Read the model definition and answer for the solid it produces. Units are mm, in the model's axes. Face numbers are marked on the shaded views. A direction names the side the tool comes from. Give positions to 0.01 mm unless a question says otherwise; leave off trailing zeros. Write each loop counter-clockwise with the first axis right and the second up, starting at its lowest first coordinate (ties: lowest second). Pieces come first, ordered by that corner, then holes. Notation, with made-up numbers: M 61,23 L 93,23 A18 ccw 93,43 Z; hole C 89,78 d5. An arc over 180 degrees is marked long. Use a Markdown table: item, result. Add a question column.
Item 1: A cutting plane is placed at B-B on x = 2506.5. Determine the outline of the cut face in (y, z).
Item 2: A cutting plane is placed at A-A on z = 6. Determine the outline of the cut face in (x, y), then the cut area to 3 significant figures.
Item 3: A cutting plane is placed at C-C on y = -484. Determine the outline of the cut face in (x, z), then the cut area to 3 significant figures.
Item 4: For the marked faces 1 and 2, determine the directions among +Z, -Z, +X, -X, +Y, -Y from which every point of the face is accessible in a straight line to the end or side of a thin tool.
Item 5: Consider probe 1 along Y at (x, z) = (2485, -14); probe 2 along X at (y, z) = (-494.5, 29.5). Determine where each line is inside the solid, lowest interval first. Write a range as [from, to].
Item 6: Given P1, Ø3, axis at y = -470, z = 35.5, coming from the -X side, flat-ended and moving along its own axis, determine where the tip first touches the part or whether it passes through.
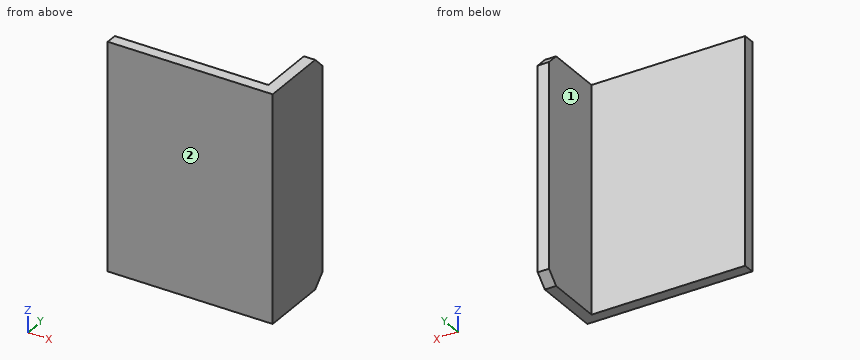
Autodesk Inventor part; units mm, degrees
ref_plane "YZ Plane" through (0, 0, 0) normal (1, 0, 0) x (0, 1, 0)
ref_plane "XZ Plane" through (0, 0, 0) normal (0, 1, 0) x (-1, 0, 0)
ref_plane "XY Plane" through (0, 0, 0) normal (0, 0, 1) x (1, 0, 0)
sketch "Sketch1" plane through (0, 0, 0) normal (0, 0, 1) x (1, 0, 0)
  line L0 (2530.6901, -554.9334) -> (2513.6901, -554.9334)
  line L1 (2513.6901, -554.9334) -> (2445.6901, -499.9334)
  line L2 (2518.6901, -464.9334) -> (2518.6901, -499.9334)
  line L3 (2513.6901, -464.9334) -> (2518.6901, -464.9334)
  line L4 (2518.6901, -499.9334) -> (2445.6901, -499.9334)
  line L5 (2445.6901, -499.9334) -> (2445.6901, -494.9334)
  line L6 (2445.6901, -494.9334) -> (2513.6901, -494.9334)
  line L7 (2513.6901, -494.9334) -> (2513.6901, -464.9334)
  line L8 (2523.6901, -464.9334) -> (2535.6901, -505.2758)
  arc A0 (2530.6901, -554.9334) -> (2535.6901, -554.9334) centre (2533.1901, -550.6033) ccw
  line L9 (2523.6901, -464.9334) -> (2518.6901, -464.9334)
  line L10 (2535.6901, -554.9334) -> (2535.6901, -505.2758)
  arc A1 (2530.6901, -554.9334) -> (2535.6901, -554.9334) centre (2533.1901, -550.6033) ccw
  line L11 (2517.6901, -494.9334) -> (1996.6901, -494.9334)
  point P0 (0, 0)
  dimension "d5" = 5
  dimension "d6" = 35
extrude "Extrusion1" add sketch "Sketch1" along normal mid plane 100 contours L5 L6 L7 L3 L2 L4
chamfer "Chamfer1" distance 5 angle 45 2 edges at (2516.1901, -464.9334, 50) (2516.1901, -464.9334, -50)
properties part number "ADSK-MH-10040" material "Steel, Mild"
Filled in:
| question | item | result |
|---|---|---|
| 1 | outline | M -499.93,-50 L -494.93,-50 L -494.93,50 L -499.93,50 Z |
| 2 | outline | M 2445.69,-499.93 L 2518.69,-499.93 L 2518.69,-464.93 L 2513.69,-464.93 L 2513.69,-494.93 L 2445.69,-494.93 Z |
| 2 | area | 515 mm² |
| 3 | outline | M 2513.69,-50 L 2518.69,-50 L 2518.69,50 L 2513.69,50 Z |
| 3 | area | 500 mm² |
| 4 | face 1 | +Z, -Z, -X, +Y |
| 4 | face 2 | +Z, -Z, +X, -X, -Y |
| 5 | probe 1 | [-499.93, -494.93] |
| 5 | probe 2 | [2513.69, 2518.69] |
| 6 | P1 | x = 2513.69 |
